Job drawing, mm, ordinate dimensions from the low corner. One solid piece. A direction names the side the tool comes from. Coordinates: 2 decimals unless noted, no trailing zeros. Write each loop counter-clockwise with the first axis right and the second up, starting at its lowest first coordinate (ties: lowest second). Pieces come first, ordered by that corner, then holes. Notation, with made-up numbers: (32.25, 7.25) -> (53.25, 7.25) arc R26 cw to (53.25, 43.25) -> close; hole circle Ø11 at (-13.75, 13). An arc over 180 degrees is marked (long way). Answer as a JSON object with one key per item and string values. Group by question number.
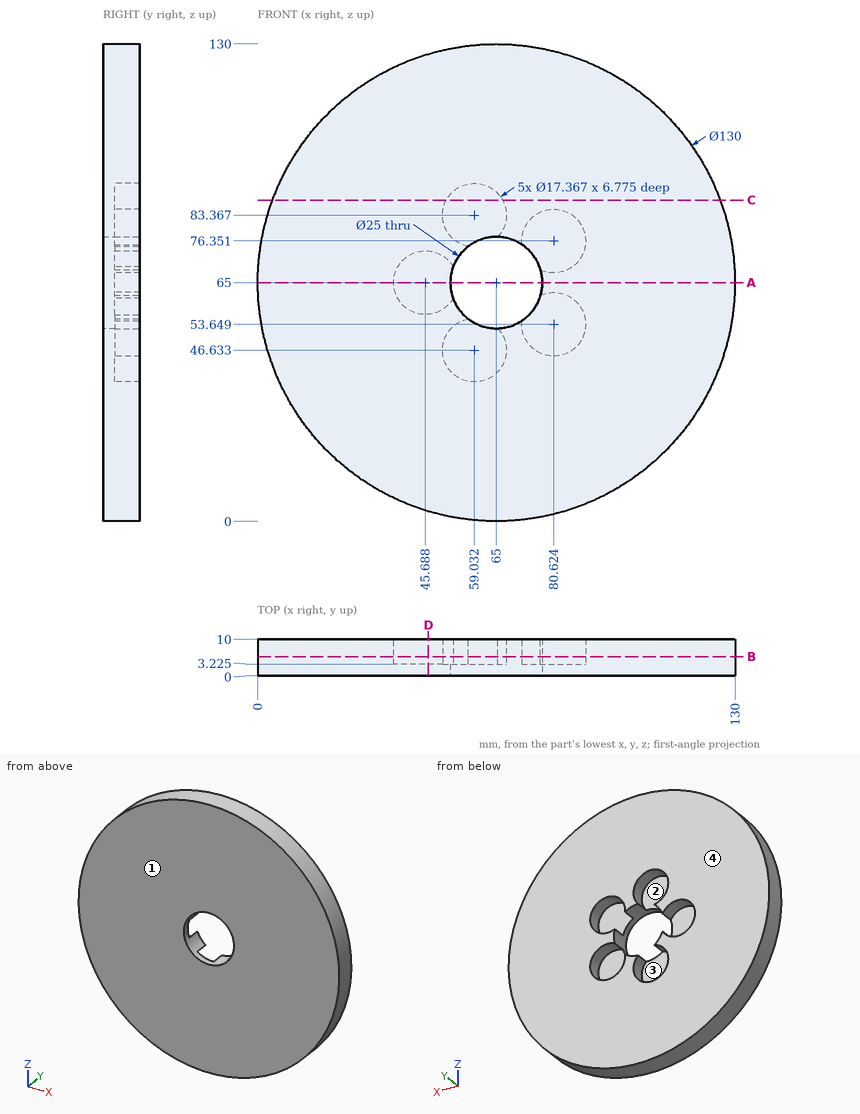
(1) Wall check: probe 1 along X at (y, z) = (7, 75.5) (1 decimal); probe 2 along Z at (x, y) = (64.5, 3); probe 3 along X at (y, z) = (3.5, 80.5) (1 decimal). Give the ranges that are in metal, low to high.
(2) Pull direction X, two halves, no side cores. Call the marked faces 3 and 4: released by +X, released by -X, zero draft, split by the parting line, or undercut.
(3) Cut at A-A on z = 65. List the corners of the cut face in (x, y) (1 decimal).
(4) Cut at B-B on y = 5.25. List the corners of the cut face in (x, z).
(5) Pin check, flat tips, straight feed: pin 1 (5 mm diameter, centred on x = 24.5, y = 2.5, fed in from +Z) (1 decimal); pin 2 (14 mm diameter, centred on x = 79.5, z = 77, fed in from +Y) (3 decimals); pin 3 (6 mm diameter, centred on y = 7, z = 66.5, fed in from -X); pin 4 (22.5 mm diameter, centred on x = 65, z = 65, fed in from -Y). Stop position of each tip, or through.
(6) Cut at D-D on x = 46.5. List the corners of the cut face in (y, z) (1 decimal), plus the area to 3 significant figures.
(7) Cut at C-C on z = 87.5. List the corners of the cut face in (x, y) (1 decimal).
(8) 3-axis set-ups, long thin cutter, end or side, ignore diameter. For the marked faces 1 and 2: which of +Z, -Z, +X, -X, +Y, -Y reach the whole face in a straight line?
Results found:
{
 "1": {"probe 1": "x = 0.9 to 55.4, 71.8 to 72, 89.3 to 129.1", "probe 2": "z = 0 to 52.51, 77.49 to 130", "probe 3": "x = 1.9 to 50.8, 67.2 to 73, 88.3 to 128.1"},
 "2": {"face 3": "undercut", "face 4": "zero draft"},
 "3": {"outline": "(0, 0) -> (52.5, 0) -> (52.5, 3.2) -> (37, 3.2) -> (37, 10) -> (0, 10) -> close; (77.5, 0) -> (130, 0) -> (130, 10) -> (77.5, 10) -> close"},
 "4": {"outline": "circle Ø130 at (65, 65); hole (53.25, 60.73) arc R12.5 ccw to (57.31, 55.14) arc R8.68 ccw (long way) to (65.43, 52.51) arc R12.5 ccw to (72, 54.64) arc R8.68 ccw (long way) to (77.01, 61.55) arc R12.5 ccw to (77.01, 68.45) arc R8.68 ccw (long way) to (72, 75.36) arc R12.5 ccw to (65.43, 77.49) arc R8.68 ccw (long way) to (57.31, 74.86) arc R12.5 ccw to (53.25, 69.27) arc R8.68 ccw (long way) to start"},
 "5": {"pin 1": "stops at z = 117.7", "pin 2": "stops at y = 3.225", "pin 3": "stops at x = 0", "pin 4": "passes through"},
 "6": {"outline": "(0, 2.7) -> (10, 2.7) -> (10, 56.4) -> (3.2, 56.4) -> (3.2, 73.6) -> (10, 73.6) -> (10, 127.3) -> (0, 127.3) -> close", "area": "1,130 mm²"},
 "7": {"outline": "(4, 0) -> (126, 0) -> (126, 10) -> (66.7, 10) -> (66.7, 3.2) -> (51.4, 3.2) -> (51.4, 10) -> (4, 10) -> close"},
 "8": {"face 1": "+Z, -Z, +X, -X, -Y", "face 2": "+Y"}
}
